from build123d import *

# Parameters (mm, degrees)
IZIM1_R                     = 2.5
Y_KSEKLIK_EKSTR_ZYON1_DEPTH = 2


with BuildPart() as part:
    # Çizim1 → Yükseklik-Ekstrüzyon1 (new body)
    with BuildSketch(Plane(origin=(0, 0, 0), x_dir=(1, 0, 0), z_dir=(0, 1, 0))):
        with BuildLine():
            Line((-18.05, 10), (18.05, 10))
            ThreePointArc((18.05, 10), (28.05, 0), (18.05, -10))
            Line((18.05, -10), (-18.05, -10))
            ThreePointArc((-18.05, -10), (-28.05, 0), (-18.05, 10))
        make_face()
        with Locations(Location((-18.05, 0, 0), (0, 0, 270))):
            Circle(IZIM1_R, mode=Mode.SUBTRACT)
        with Locations(Location((18.05, 0, 0), (0, 0, 270))):
            Circle(IZIM1_R, mode=Mode.SUBTRACT)
    extrude(amount=Y_KSEKLIK_EKSTR_ZYON1_DEPTH)


solid = part.part
Geometry: final body of the model. Coordinates: model frame, mm. Give positions to 0.01 mm unless a question says otherwise; leave off trailing zeros. Loops run counter-clockwise (first coordinate to the right, second up) from the corner with the lowest first, then second, coordinate; pieces in that order, holes last. Notation, with made-up numbers: (3, -29.75) - (26, -29.75) arc R33 ccw to (26, 8.25) - close; hole circle Ø8 at (-26, 35.25). An arc over 180 degrees is marked (long way). Answer as CSV lines item,"result". Start each with the question number.
1. Section A-A, the plane z = 0. Return loops of the section in (x, y).
2. Pin query (flat end, axial travel): P1, Ø1, axis at y = 1, z = -5.5, coming from the +X side. Return the tip coordinate at first contact, or that it passes through.
3. Draft query along X for faces 1 (the face through (-28.048, 0.986, 0.22)), 2 (the face through (-20.5, 1, -0.5)), 3 (the face through (0, 0, 0)). Return one class per face: released by +X, released by -X, zero draft, split by the parting line, or undercut.
4. Section C-C, the plane y = 0.9. Return loops of the section in (x, z).
5. Section B-B, the plane x = 17.5. Return loops of the section in (y, z).
6. Section D-D, the plane z = 8. Return loops of the section in (x, y).
7. Ray query, L1, parallel to X at y = 1.45, z = 0; L2, parallel to X at y = 0.35, z = -2; L3, parallel to X at y = 1.45, z = 6.25. Return the intervals inside material, ascending.
Answers:
1,outline,"(-28.05, 0) - (-20.55, 0) - (-20.55, 2) - (-28.05, 2) - close; (-15.55, 0) - (15.55, 0) - (15.55, 2) - (-15.55, 2) - close; (20.55, 0) - (28.05, 0) - (28.05, 2) - (20.55, 2) - close"
2,P1,"stops at x = 26.71"
3,face 1,"released by -X"
3,face 2,"undercut"
3,face 3,"zero draft"
4,outline,"(-18.05, -10) - (18.05, -10) arc R10 ccw to (18.05, 10) - (-18.05, 10) arc R10 ccw to start; hole circle Ø5 at (-18.05, 0); hole circle Ø5 at (18.05, 0)"
5,outline,"(0, -10) - (2, -10) - (2, -2.44) - (0, -2.44) - close; (0, 2.44) - (2, 2.44) - (2, 10) - (0, 10) - close"
6,outline,"(-24.05, 0) - (24.05, 0) - (24.05, 2) - (-24.05, 2) - close"
7,L1,"x = -28.05 to -20.55, -15.55 to 15.55, 20.55 to 28.05"
7,L2,"x = -27.85 to -19.55, -16.55 to 16.55, 19.55 to 27.85"
7,L3,"x = -25.86 to 25.86"
